Part model, mm, in its own coordinate system. Face numbers are marked on the shaded views. A direction names the side the tool comes from. Coordinates: 2 decimals unless noted, no trailing zeros. Loops run counter-clockwise (first coordinate to the right, second up) from the corner with the lowest first, then second, coordinate; pieces in that order, holes last. Notation, with made-up numbers: M 81,-36.5 L 137,-36.5 A13 cw 137,-20.5 Z; hole C -25,56.5 d6. An arc over 180 degrees is marked long. Use a Markdown table: item, result. Add a question column.
1) Band-saw the part on C-C (x = 0). List the corners of the cut face in (y, z), plus the area to 3 significant figures.
2) Band-saw the part on A-A (y = 5). List the corners of the cut face in (x, z).
3) Band-saw the part on D-D (x = 2.4). List the corners of the cut face in (y, z), plus the area to 3 significant figures.
4) Pin check, flat tips, straight feed: pin 1 Ø3 at (x, y) = (0.5, 4.5) entering from -Z; pin 2 Ø3 at (x, z) = (1.5, 5.5) entering from +Y; pin 3 Ø3 at (x, y) = (0, 3.5) entering from +Z; pin 4 Ø2 at (x, z) = (0, 4.75) entering from +Y. Stop position of each tip, or through.
5) Pull direction X, two halves, no side cores. Call the marked faces 1, 2, 3 and 4: released by +X, released by -X, zero draft, split by the parting line, or undercut.
6) Wall check: probe 1 along Z at (x, y) = (-1.7, 1.5); probe 2 along X at (y, z) = (5, -1.1); probe 3 along Y at (x, z) = (0, 1.25). Give the ranges that are in metal, low to high. Write a range as from..to.
7) Band-saw the part on B-B (z = -4.75). List the corners of the cut face in (x, y).
8) Tool access for the marked faces 5, 6 and 7: list every direction of +Z, -Z, +X, -X, +Y, -Y with a clear straight run to the whole face (end or side of a thin tool).
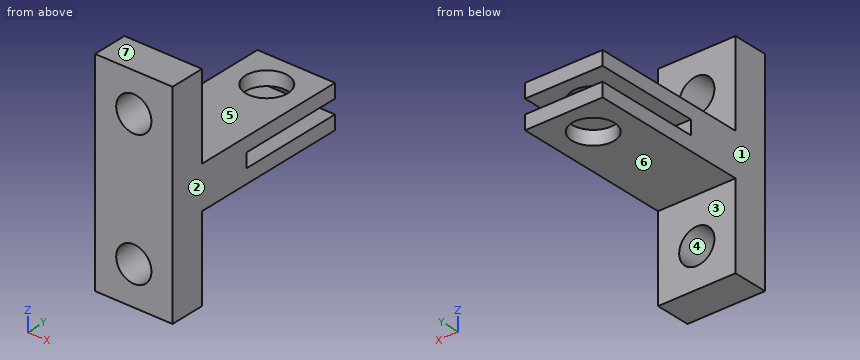
from build123d import *

# Parameters (mm, degrees)
BOSS_EXTRUDE1_DEPTH     = 2.75
SKETCH2_R               = 1.25
CUT_EXTRUDE1_DEPTH      = 14.838442831
CUT_EXTRUDE2_DEPTH      = 11.9573035
CUT_EXTRUDE2_DEPTH_BACK = 11.9573035
SKETCH4_R               = 1.5


with BuildPart() as part:
    # Sketch1 → Boss-Extrude1 (new, symmetric)
    with BuildSketch(Plane(origin=(0, 0, 0), x_dir=(0, 0, -1), z_dir=(1, 0, 0))):
        Polygon((-0.5, 7.5), (-0.5, 0), (0.5, 0), (0.5, 7.5), (1.5, 7.5), (1.5, -3.8), (7.5, -3.8), (7.5, -6.3), (-7.5, -6.3), (-7.5, -3.8), (-1.5, -3.8), (-1.5, 7.5), align=None)
    extrude(amount=BOSS_EXTRUDE1_DEPTH, both=True)

    # Sketch2 → Cut-Extrude1 (cut, through all)
    with BuildSketch(Plane(origin=(0, -3.8, 0), x_dir=(1, 0, 0), z_dir=(0, 1, 0))):
        with Locations(Location((0, -4.75, 0), (0, 0, 270))):
            Circle(SKETCH2_R)
        with Locations(Location((0, 4.75, 0), (0, 0, 90))):
            Circle(SKETCH2_R)
    extrude(amount=-CUT_EXTRUDE1_DEPTH, mode=Mode.SUBTRACT)

    # Sketch4 → Cut-Extrude2 (cut, two sides: drawn at the far end of the back side and taken through both)
    with BuildSketch(Plane.XY.offset(-CUT_EXTRUDE2_DEPTH_BACK)):
        with Locations(Location((0, 5, 0), (0, 0, 270))):
            Circle(SKETCH4_R)
    extrude(amount=CUT_EXTRUDE2_DEPTH + CUT_EXTRUDE2_DEPTH_BACK, mode=Mode.SUBTRACT)


solid = part.part
Entries:
| question | item | result |
|---|---|---|
| 1 | outline | M -6.3,-7.5 L -3.8,-7.5 L -3.8,-6 L -6.3,-6 Z; M -6.3,-3.5 L -3.8,-3.5 L -3.8,-1.5 L 3.5,-1.5 L 3.5,-0.5 L 0,-0.5 L 0,0.5 L 3.5,0.5 L 3.5,1.5 L -3.8,1.5 L -3.8,3.5 L -6.3,3.5 Z; M -6.3,6 L -3.8,6 L -3.8,7.5 L -6.3,7.5 Z; M 6.5,-1.5 L 7.5,-1.5 L 7.5,-0.5 L 6.5,-0.5 Z; M 6.5,0.5 L 7.5,0.5 L 7.5,1.5 L 6.5,1.5 Z |
| 1 | area | 45.4 mm2 |
| 2 | outline | M -2.75,-1.5 L -1.5,-1.5 L -1.5,-0.5 L -2.75,-0.5 Z; M -2.75,0.5 L -1.5,0.5 L -1.5,1.5 L -2.75,1.5 Z; M 1.5,-1.5 L 2.75,-1.5 L 2.75,-0.5 L 1.5,-0.5 Z; M 1.5,0.5 L 2.75,0.5 L 2.75,1.5 L 1.5,1.5 Z |
| 3 | outline | M -6.3,-7.5 L -3.8,-7.5 L -3.8,-1.5 L 7.5,-1.5 L 7.5,-0.5 L 0,-0.5 L 0,0.5 L 7.5,0.5 L 7.5,1.5 L -3.8,1.5 L -3.8,7.5 L -6.3,7.5 Z |
| 3 | area | 63.9 mm2 |
| 4 | pin 1 | z = -1.5 |
| 4 | pin 2 | y = -3.8 |
| 4 | pin 3 | z = 1.5 |
| 4 | pin 4 | through |
| 5 | face 1 | released by -X |
| 5 | face 2 | released by +X |
| 5 | face 3 | zero draft |
| 5 | face 4 | undercut |
| 6 | probe 1 | -1.5..-0.5, 0.5..1.5 |
| 6 | probe 2 | -2.75..-1.5, 1.5..2.75 |
| 6 | probe 3 | -6.3..3.5, 6.5..7.5 |
| 7 | outline | M -2.75,-6.3 L -1.25,-6.3 L -1.25,-3.8 L -2.75,-3.8 Z; M 1.25,-6.3 L 2.75,-6.3 L 2.75,-3.8 L 1.25,-3.8 Z |
| 8 | face 5 | +Z, +X, -X, +Y |
| 8 | face 6 | -Z, +X, -X, +Y |
| 8 | face 7 | +Z, +X, -X, +Y, -Y |
